from build123d import *

# Parameters (mm, degrees)
SKETCH1_W           = 82.55
SKETCH1_H           = 114.3
BOSS_EXTRUDE1_DEPTH = 27.94
FILLET1_R           = 2.54
SHELL2_START        = -38.735
SHELL2_OUTLINE_W    = 25.4
SHELL2_OUTLINE_H    = 109.22
SHELL2_DEPTH        = 77.47
SKETCH2_W           = 55.88
SKETCH2_H           = 5.08
BOSS_EXTRUDE2_DEPTH = 19.05
CUT_EXTRUDE1_REACH  = 106.217
SKETCH3_R           = 1.75
CUT_EXTRUDE2_REACH  = 126.695
SKETCH4_R           = 6.35
CUT_EXTRUDE3_REACH  = 126.695
SKETCH5_W           = 19.05
SKETCH5_H           = 12.7
SKETCH6_W           = 38.735
SKETCH6_H           = 2.54
SKETCH6_H_2         = 1.27
SKETCH6_W_2         = 1.27
CUT_EXTRUDE4_DEPTH  = 111.76


# Read off the part's stored shape, not the designer's step: Shell2
with BuildPart() as part:
    # Sketch1 → Boss-Extrude1 (new body)
    with BuildSketch(Plane(origin=(0, 0, 0), x_dir=(1, 0, 0), z_dir=(0, 1, 0))):
        Rectangle(SKETCH1_W, SKETCH1_H)
    extrude(amount=BOSS_EXTRUDE1_DEPTH)

    # Fillet1
    fillet1_edges = [part.edges().sort_by_distance(p)[0] for p in [
        (-41.275, 27.94, 0),
        (0, 27.94, 57.15),
        (41.275, 27.94, 0),
        (0, 0, 57.15),
        (-41.275, 0, 0),
        (0, 0, -57.15),
        (41.275, 0, 0),
        (41.275, 13.97, 57.15),
        (-41.275, 13.97, 57.15),
        (-41.275, 13.97, -57.15),
        (41.275, 13.97, -57.15),
        (0, 27.94, -57.15),
    ]]
    fillet(fillet1_edges, radius=FILLET1_R)

    # Shell2 outline → Shell2 (cut)
    with BuildSketch(Plane.YZ.offset(SHELL2_START)):
        with Locations((15.24, 0)):
            Rectangle(SHELL2_OUTLINE_W, SHELL2_OUTLINE_H)
    extrude(amount=SHELL2_DEPTH, mode=Mode.SUBTRACT)

    # Sketch2 → Boss-Extrude2 (add)
    with BuildSketch(Plane(origin=(0, 2.54, 0), x_dir=(1, 0, 0), z_dir=(0, 1, 0))):
        with Locations((-10.795, -24.13)):
            Rectangle(SKETCH2_W, SKETCH2_H)
        with Locations((10.795, 24.13)):
            Rectangle(SKETCH2_W, SKETCH2_H)
    extrude(amount=BOSS_EXTRUDE2_DEPTH)

    # Sketch3 → Cut-Extrude1 (cut, up to next)
    with BuildSketch(Plane.ZY.offset(41.275), mode=Mode.PRIVATE) as cut_extrude1_sk1:
        with Locations((13.97, 13.97)):
            Circle(SKETCH3_R)
    cut_extrude1_tool1 = extrude(cut_extrude1_sk1.sketch, amount=-CUT_EXTRUDE1_REACH, mode=Mode.PRIVATE) & part.part
    add(cut_extrude1_tool1.solids().sort_by_distance((-41.275, 13.97, 13.97))[0], mode=Mode.SUBTRACT)

    # Sketch4 → Cut-Extrude2 (cut, up to next)
    with BuildSketch(Plane.XY.offset(57.15), mode=Mode.PRIVATE) as cut_extrude2_sk1:
        with Locations((-28.575, 13.97)):
            Circle(SKETCH4_R)
    cut_extrude2_tool1 = extrude(cut_extrude2_sk1.sketch, amount=-CUT_EXTRUDE2_REACH, mode=Mode.PRIVATE) & part.part
    add(cut_extrude2_tool1.solids().sort_by_distance((-28.575, 13.97, 57.15))[0], mode=Mode.SUBTRACT)

    # Sketch5 → Cut-Extrude3 (cut, up to next)
    with BuildSketch(Plane(origin=(0, 0, -57.15), x_dir=(-1, 0, 0), z_dir=(0, 0, -1)), mode=Mode.PRIVATE) as cut_extrude3_sk1:
        with Locations((-22.225, 13.97)):
            Rectangle(SKETCH5_W, SKETCH5_H)
    cut_extrude3_tool1 = extrude(cut_extrude3_sk1.sketch, amount=-CUT_EXTRUDE3_REACH, mode=Mode.PRIVATE) & part.part
    add(cut_extrude3_tool1.solids().sort_by_distance((22.225, 13.97, -57.15))[0], mode=Mode.SUBTRACT)

    # Sketch6 → Cut-Extrude4 (cut)
    with BuildSketch(Plane(origin=(0, 0, -57.15), x_dir=(-1, 0, 0), z_dir=(0, 0, -1))):
        with Locations((-19.3675, 26.67)):
            Rectangle(SKETCH6_W, SKETCH6_H)
        with Locations((-19.3675, 24.765)):
            Rectangle(SKETCH6_W, SKETCH6_H_2)
        with Locations((-39.37, 24.765)):
            Rectangle(SKETCH6_W_2, SKETCH6_H_2)
        with Locations((39.37, 24.765)):
            Rectangle(SKETCH6_W_2, SKETCH6_H_2)
        with Locations((19.3675, 26.67)):
            Rectangle(SKETCH6_W, SKETCH6_H)
        with Locations((19.3675, 24.765)):
            Rectangle(SKETCH6_W, SKETCH6_H_2)
    extrude(amount=-CUT_EXTRUDE4_DEPTH, mode=Mode.SUBTRACT)


solid = part.part
Geometry check sheet. Reference: the model listing, model coordinates, mm. A direction names the side the tool comes from. Give positions to 0.01 mm unless a question says otherwise; leave off trailing zeros. Order: outer loops, then holes, each group sorted by start corner. A loop starts at its lowest first (then second) coordinate and runs counter-clockwise, first axis right, second up. Notation, with made-up numbers: (54, -6.75) - (66, -6.75) arc R34 cw to (66, 28.25) - close; hole circle Ø3 at (50, 53.25). An arc over 180 degrees is marked (long way). Use one line per item in the form item = value.
1) Sectioned sample at B-B (z = 13.97). Record the boundary of the cut face in (x, y) (3 decimals), and give its area (3 significant figures).
Working result:
outline = (-41.275, 2.54) arc R2.54 ccw to (-38.735, 0) - (38.735, 0) arc R2.54 ccw to (41.275, 2.54) - (41.275, 25.4) arc R2.54 ccw to (38.735, 27.94) - (38.735, 25.4) - (40.005, 25.4) - (40.005, 24.13) - (38.735, 24.13) - (38.735, 2.54) - (-38.735, 2.54) - (-38.735, 12.22) - (-41.275, 12.22) - close; (-41.275, 15.72) - (-38.735, 15.72) - (-38.735, 24.13) - (-40.005, 24.13) - (-40.005, 25.4) - (-38.735, 25.4) - (-38.735, 27.94) arc R2.54 ccw to (-41.275, 25.4) - close
area = 321 mm^2
2) Sectioned sample at A-A (x = 23.5). Record the boundary of the cut face in (y, z), and give its area (3 significant figures).
Working result:
outline = (0, -54.61) arc R2.54 ccw to (2.54, -57.15) - (7.62, -57.15) - (7.62, -54.61) - (2.54, -54.61) - (2.54, -26.67) - (21.59, -26.67) - (21.59, -21.59) - (2.54, -21.59) - (2.54, 54.61) - (27.94, 54.61) arc R2.54 ccw to (25.4, 57.15) - (2.54, 57.15) arc R2.54 ccw to (0, 54.61) - close; (20.32, -57.15) - (24.13, -57.15) - (24.13, -54.61) - (20.32, -54.61) - close
area = 470 mm^2
3) Draft check along X on faces 3 (the face through (0.542, 0.764, -56.426)), 4 (the face through (-17.145, 12, -24)), 5 (the face through (-40.551, 14.13, 56.386)). Enter one of: released by +X, released by -X, zero draft, split by the parting line, or undercut.
Working result:
face_3 = zero draft
face_4 = undercut
face_5 = released by -X
4) Access from +Z, -Z, +X, -X, +Y, -Y to the whole of each face (thin tool, end or side, straight path). Record for faces 1 (the face through (40.511, 14.13, 56.426)), 2 (the face through (-11, 12, 26.67)).
Working result:
face_1 = +Z, +X, +Y, -Y
face_2 = +Y
5) Material ranges on probe 1 along Z at (x, y) = (-29.5, 4.25); probe 2 along Z at (x, y) = (18.5, 21); probe 3 along Z at (x, y) = (6.5, 10.5), recorded low to high. Write a range as from..to.
Working result:
probe_1 = -57.15..-54.61, 21.59..26.67, 54.61..57.15
probe_2 = -57.15..-54.61, -26.67..-21.59, 54.61..57.15
probe_3 = -57.15..-54.61, -26.67..-21.59, 21.59..26.67, 54.61..57.15
6) Sectioned sample at D-D (x = 11). Record the boundary of the cut face in (y, z), and give its area (3 significant figures).
Working result:
outline = (0, -54.61) arc R2.54 ccw to (2.54, -57.15) - (24.13, -57.15) - (24.13, -54.61) - (2.54, -54.61) - (2.54, -26.67) - (21.59, -26.67) - (21.59, -21.59) - (2.54, -21.59) - (2.54, 21.59) - (21.59, 21.59) - (21.59, 26.67) - (2.54, 26.67) - (2.54, 54.61) - (27.94, 54.61) arc R2.54 ccw to (25.4, 57.15) - (2.54, 57.15) arc R2.54 ccw to (0, 54.61) - close
area = 599 mm^2
7) Sectioned sample at C-C (y = 13.97). Count the separate pieces of the cut face and the enclosed holes in it, and give its area (3 significant figures).
Working result:
separate_pieces = 3
enclosed_holes = 0
area = 1,450 mm^2
8) Depth check by flat-ended pin: pin 1 Ø1.3 at (y, z) = (26.5, 9.5) entering from -X; pin 2 Ø3 at (x, z) = (22.5, -55.5) entering from +Y; pin 3 Ø1 at (x, z) = (-31.5, -31.5) entering from +Y. Enter the tip coordinate at first touch or a pass-through.
Working result:
pin_1 = -41.23
pin_2 = 24.13
pin_3 = 2.54
